The model under review builds one solid part; all positions refer to its coordinate system, in mm. Coordinates: 2 decimals unless noted, no trailing zeros. Loops run counter-clockwise (first coordinate to the right, second up) from the corner with the lowest first, then second, coordinate; pieces in that order, holes last. Notation, with made-up numbers: (76.5, 12.25) - (128.5, 12.25) arc R19 cw to (128.5, 39.25) - close; hole circle Ø3 at (9.5, 41). An arc over 180 degrees is marked (long way). One line per item, written item: value. Start each with the question number.
1. To check wall thickness, follow line 1 (Y direction, x = 1.7, z = 34.5); line 2 (Y direction, x = 3.05, z = 24.75); line 3 (Y direction, x = 2.85, z = 3). State the ranges of each line that lie inside material, in increasing order.
2. We need section B-B, the plane y = -15. Give the boundary of the cut face in (x, z), then the cut area to 3 significant figures.
3. We need section D-D, the plane z = -1. Give the boundary of the cut face in (x, y).
4. Insertion check: P1, Ø1.5, axis at y = 1.5, z = 27, coming from the -X side. The pin has a flat end and moves straight along its axis. Give the tip position at first contact, or say it passes through.
5. We need section A-A, the plane z = -24.75. Give the boundary of the cut face in (x, y).
6. We need section C-C, the plane y = 5. Give the boundary of the cut face in (x, z), then the cut area to 3 significant figures.
from build123d import *

# Parameters (mm, degrees)
SKETCH_1_W          = 79
SKETCH_1_H          = 40
SKETCH_1_R          = 2.1
SKETCH_1_W_2        = 40.5
SKETCH_1_H_2        = 20.5
EXTRUDE_1_DEPTH     = 4
FILLET_1_R          = 4
SKETCH_2_R          = 1.5
CUT_EXTRUDE_1_DEPTH = 10
FILLET_2_R          = 2


with BuildPart() as part:
    # 草图1 → 凸台-拉伸1 (new body)
    with BuildSketch(Plane(origin=(0, 0, 0), x_dir=(0, 0, -1), z_dir=(1, 0, 0))):
        Rectangle(SKETCH_1_W, SKETCH_1_H)
        with Locations((-34.5, 15)):
            Circle(SKETCH_1_R, mode=Mode.SUBTRACT)
        with Locations((-34.5, -15)):
            Circle(SKETCH_1_R, mode=Mode.SUBTRACT)
        with Locations((-24.75, -5)):
            Circle(SKETCH_1_R, mode=Mode.SUBTRACT)
        with Locations((-24.75, 5)):
            Circle(SKETCH_1_R, mode=Mode.SUBTRACT)
        with Locations((24.75, 5)):
            Circle(SKETCH_1_R, mode=Mode.SUBTRACT)
        with Locations((24.75, -5)):
            Circle(SKETCH_1_R, mode=Mode.SUBTRACT)
        with Locations((34.5, 15)):
            Circle(SKETCH_1_R, mode=Mode.SUBTRACT)
        with Locations((34.5, -15)):
            Circle(SKETCH_1_R, mode=Mode.SUBTRACT)
        Rectangle(SKETCH_1_W_2, SKETCH_1_H_2, mode=Mode.SUBTRACT)
    extrude(amount=EXTRUDE_1_DEPTH)

    # 圆角1
    fillet_1_edges = [part.edges().sort_by_distance(p)[0] for p in [
        (2, -20, -39.5),
        (2, -20, 39.5),
        (2, 20, 39.5),
        (2, 20, -39.5),
    ]]
    fillet(fillet_1_edges, radius=FILLET_1_R)

    # 草图2 → 切除-拉伸1 (cut)
    with BuildSketch(Plane(origin=(4, 0, 0), x_dir=(0, 0, -1), z_dir=(1, 0, 0))):
        with Locations((-20.25, 10.25)):
            Circle(SKETCH_2_R)
        with Locations((-20.25, -10.25)):
            Circle(SKETCH_2_R)
        with Locations((20.25, -10.239026698)):
            Circle(SKETCH_2_R)
        with Locations((20.25, 10.25)):
            Circle(SKETCH_2_R)
    extrude(amount=-CUT_EXTRUDE_1_DEPTH, mode=Mode.SUBTRACT)

    # 圆角2
    fillet_2_edges = [part.edges().sort_by_distance(p)[0] for p in [
        (2, -10.25, 18.75),
        (2, 8.75, -20.25),
        (2, -10.25, -18.750040138),
        (2, -8.75, 20.25),
        (2, 8.75, 20.25),
        (2, 10.25, 18.75),
        (2, 10.25, -18.75),
        (2, -8.739026698, -20.25),
    ]]
    fillet(fillet_2_edges, radius=FILLET_2_R)


solid = part.part
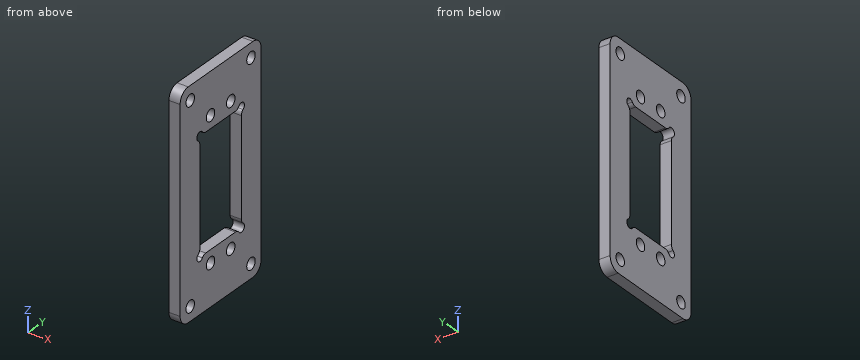
Findings below:
1. line 1: -20 to -17.1, -12.9 to 12.9, 17.1 to 20
1. line 2: -20 to -7.1, -2.9 to 2.9, 7.1 to 20
1. line 3: -20 to -10.25, 10.25 to 20
2. outline: (0, -39.5) - (4, -39.5) - (4, -36.6) - (0, -36.6) - close; (0, -32.4) - (4, -32.4) - (4, 32.4) - (0, 32.4) - close; (0, 36.6) - (4, 36.6) - (4, 39.5) - (0, 39.5) - close
2. area: 282 mm2
3. outline: (0, -20) - (4, -20) - (4, -10.25) - (0, -10.25) - close; (0, 10.25) - (4, 10.25) - (4, 20) - (0, 20) - close
4. P1: x = 0
5. outline: (0, -20) - (4, -20) - (4, -7.1) - (0, -7.1) - close; (0, -2.9) - (4, -2.9) - (4, 2.9) - (0, 2.9) - close; (0, 7.1) - (4, 7.1) - (4, 20) - (0, 20) - close
6. outline: (0, -39.5) - (4, -39.5) - (4, -26.85) - (0, -26.85) - close; (0, -22.65) - (4, -22.65) - (4, -20.25) - (0, -20.25) - close; (0, 20.25) - (4, 20.25) - (4, 22.65) - (0, 22.65) - close; (0, 26.85) - (4, 26.85) - (4, 39.5) - (0, 39.5) - close
6. area: 120 mm2
